from build123d import *

# Parameters (mm, degrees)
SKETCH1_W           = 25.4
SKETCH1_H           = 125.4
BOSS_EXTRUDE1_DEPTH = 6.35
SKETCH2_W           = 112.7
SKETCH2_H           = 6.35
CUT_EXTRUDE1_DEPTH  = 12.7
SKETCH3_W           = 12.7
SKETCH3_H           = 6.35
CUT_EXTRUDE2_DEPTH  = 6.35
SKETCH4_W           = 8.65
SKETCH4_H           = 6.35
BOSS_EXTRUDE2_DEPTH = 12.7
SKETCH5_W           = 6.35
SKETCH5_H           = 6.35
BOSS_EXTRUDE3_DEPTH = 12.7
SKETCH6_W           = 6.35
SKETCH6_H           = 6.35
BOSS_EXTRUDE4_DEPTH = 12.7
SKETCH10_W          = 6.35
SKETCH10_H          = 6.35
CUT_EXTRUDE3_DEPTH  = 7.35


with BuildPart() as part:
    # Sketch1 → Boss-Extrude1 (new body)
    with BuildSketch(Plane(origin=(0, 0, 0), x_dir=(1, 0, 0), z_dir=(0, 1, 0))):
        Rectangle(SKETCH1_W, SKETCH1_H)
    extrude(amount=BOSS_EXTRUDE1_DEPTH)

    # Sketch2 → Cut-Extrude1 (cut)
    with BuildSketch(Plane.ZY.offset(12.7)):
        with Locations((0, 3.175)):
            Rectangle(SKETCH2_W, SKETCH2_H)
    extrude(amount=-CUT_EXTRUDE1_DEPTH, mode=Mode.SUBTRACT)

    # Sketch3 → Cut-Extrude2 (cut)
    with BuildSketch(Plane(origin=(12.7, 0, 0), x_dir=(0, 0, -1), z_dir=(1, 0, 0))):
        with Locations((0, 3.175)):
            Rectangle(SKETCH3_W, SKETCH3_H)
    extrude(amount=-CUT_EXTRUDE2_DEPTH, mode=Mode.SUBTRACT)

    # Sketch4 → Boss-Extrude2 (add)
    with BuildSketch(Plane(origin=(12.7, 0, 0), x_dir=(0, 0, -1), z_dir=(1, 0, 0))):
        with Locations((-10.675, 3.175)):
            Rectangle(SKETCH4_W, SKETCH4_H)
    boss_extrude2 = extrude(amount=BOSS_EXTRUDE2_DEPTH)

    # Mirror1: Boss-Extrude2 across plane
    add(boss_extrude2.mirror(Plane.XY))

    # Sketch5 → Boss-Extrude3 (add)
    with BuildSketch(Plane(origin=(12.7, 0, 0), x_dir=(0, 0, -1), z_dir=(1, 0, 0))):
        with Locations((46.825, 3.175)):
            Rectangle(SKETCH5_W, SKETCH5_H)
    boss_extrude3 = extrude(amount=BOSS_EXTRUDE3_DEPTH)

    # Sketch6 → Boss-Extrude4 (add)
    with BuildSketch(Plane(origin=(12.7, 0, 0), x_dir=(0, 0, -1), z_dir=(1, 0, 0))):
        with Locations((34.125, 3.175)):
            Rectangle(SKETCH6_W, SKETCH6_H)
    boss_extrude4 = extrude(amount=BOSS_EXTRUDE4_DEPTH)

    # Mirror2: Boss-Extrude3, Boss-Extrude4 across plane
    add(boss_extrude3.mirror(Plane.XY))
    add(boss_extrude4.mirror(Plane.XY))

    # Sketch10 → Cut-Extrude3 (cut, through all)
    with BuildSketch(Plane(origin=(0, 6.35, 0), x_dir=(1, 0, 0), z_dir=(0, 1, 0))):
        with Locations((-9.525, 59.525)):
            Rectangle(SKETCH10_W, SKETCH10_H)
    cut_extrude3 = extrude(amount=-CUT_EXTRUDE3_DEPTH, mode=Mode.SUBTRACT)

    # Mirror3: Cut-Extrude3 across plane
    add(cut_extrude3.mirror(Plane.XY), mode=Mode.SUBTRACT)


solid = part.part
Could you check a few things on this model? Use its own coordinates, in mm. A direction names the side the tool comes from. Give positions to 0.01 mm unless a question says otherwise; leave off trailing zeros. Order: outer loops, then holes, each group sorted by start corner. A loop starts at its lowest first (then second) coordinate and runs counter-clockwise, first axis right, second up. Notation, with made-up numbers: (33.25, -3) -> (45.25, -3) arc R23 cw to (45.25, 22) -> close; hole circle Ø3 at (-5, -10.5). An arc over 180 degrees is marked (long way). Answer in a Markdown table with one row per item. Add a question column.
Item 1: Imagine slicing it at B-B (x = 14.5). List the corners of the cut face in (y, z) for me.
Item 2: Imagine slicing it at A-A (x = 8.5). List the corners of the cut face in (y, z) for me.
Item 3: Imagine slicing it at D-D (z = -26.5). List the corners of the cut face in (x, y) for me, and give its area (3 significant figures).
Item 4: Please list where these lines run through material, in increasing order: probe 1 along Z at (x, y) = (16, 3.5); probe 2 along Z at (x, y) = (-4, 5); probe 3 along X at (y, z) = (6, -49.5).
Item 5: I'm going to push flat-ended pins straight in: P1, Ø3, axis at x = 21.5, y = 4.5, coming from the +Z side; P2, Ø1.9, axis at x = 21.5, y = 4.5, coming from the -Z side; P3, Ø3, axis at y = 3.5, z = 2, coming from the +X side. Where does each tip first touch, or does it pass through?
Item 6: For faces 4 (the flat face through (25.4, 3, 34)), 5 (the flat face through (19, 3, 15)), which set-ups out of +Z, -Z, +X, -X, +Y, -Y let a thin tool reach every point of the face, with its end or its side?
Item 7: We'd pull the mould along Z, two halves only. Please class faces 1 (the flat face through (25.4, 3, 47)), 2 (the flat face through (19, 3, -50)), 3 (the flat face through (12.7, 3, 41)): pulls with the +Z half, pulls with the -Z half, needs draft (parallel to the pull), parting line crosses it, or undercut.
Result:
| question | item | result |
|---|---|---|
| 1 | outline | (0, -50) -> (6.35, -50) -> (6.35, -43.65) -> (0, -43.65) -> close; (0, -37.3) -> (6.35, -37.3) -> (6.35, -30.95) -> (0, -30.95) -> close; (0, -15) -> (6.35, -15) -> (6.35, -6.35) -> (0, -6.35) -> close; (0, 6.35) -> (6.35, 6.35) -> (6.35, 15) -> (0, 15) -> close; (0, 30.95) -> (6.35, 30.95) -> (6.35, 37.3) -> (0, 37.3) -> close; (0, 43.65) -> (6.35, 43.65) -> (6.35, 50) -> (0, 50) -> close |
| 2 | outline | (0, -62.7) -> (6.35, -62.7) -> (6.35, -6.35) -> (0, -6.35) -> close; (0, 6.35) -> (6.35, 6.35) -> (6.35, 62.7) -> (0, 62.7) -> close |
| 3 | outline | (0, 0) -> (12.7, 0) -> (12.7, 6.35) -> (0, 6.35) -> close |
| 3 | area | 80.6 mm2 |
| 4 | probe 1 | -50 to -43.65, -37.3 to -30.95, -15 to -6.35, 6.35 to 15, 30.95 to 37.3, 43.65 to 50 |
| 4 | probe 2 | -62.7 to -56.35, 56.35 to 62.7 |
| 4 | probe 3 | 0 to 25.4 |
| 5 | P1 | z = 50 |
| 5 | P2 | z = -50 |
| 5 | P3 | x = 6.35 |
| 6 | face 4 | +Z, -Z, +X, +Y, -Y |
| 6 | face 5 | +X, +Y, -Y |
| 7 | face 1 | needs draft |
| 7 | face 2 | pulls with the -Z half |
| 7 | face 3 | undercut |
